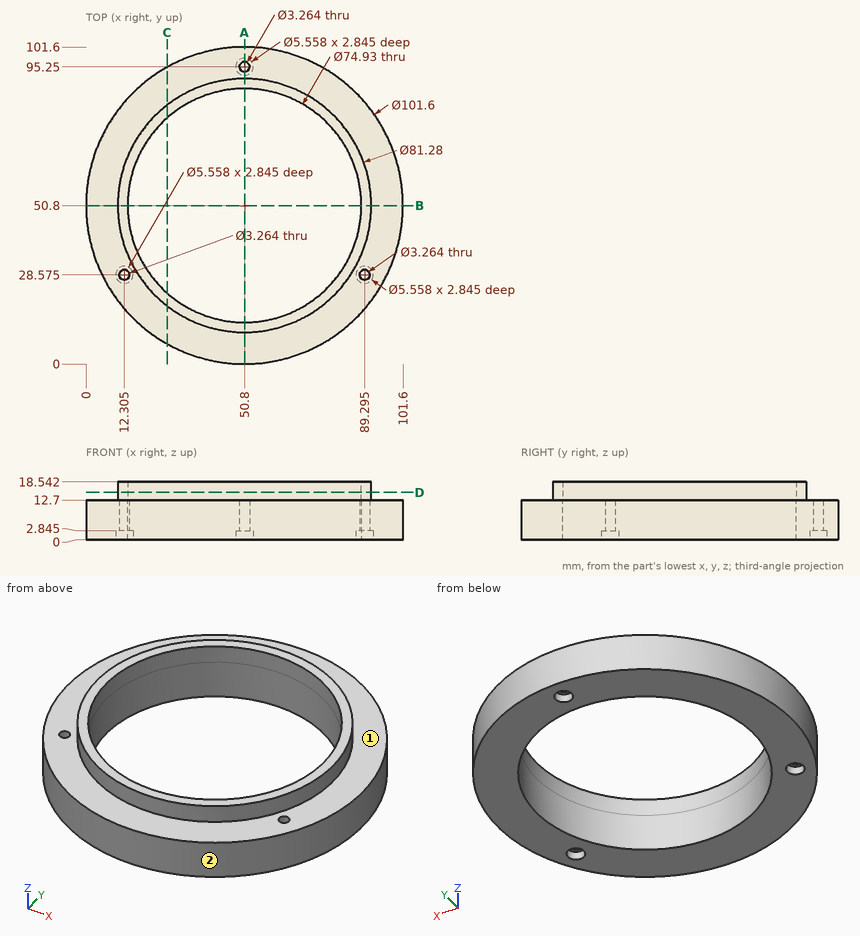
Source: three-view drawing plus pictorial views. Frame: mm from the lowest corner of the part. A direction names the side the tool comes from. Round coordinates to 2 decimals unless told otherwise and drop trailing zeros. Write each loop counter-clockwise with the first axis right and the second up, starting at its lowest first coordinate (ties: lowest second). Pieces come first, ordered by that corner, then holes. Notation, with made-up numbers: M 73,61.5 L 94,61.5 A19 ccw 94,98.5 Z; hole C -13.5,23 d6. An arc over 180 degrees is marked long. One line per item, written item: value. Start each with the question number.
Item 1: Pin query (flat end, axial travel): pin 1 (5 mm diameter, centred on y = 15.5, z = 7.5, fed in from +X); pin 2 (2 mm diameter, centred on y = 84, z = 14, fed in from +X) (1 decimal); pin 3 (4 mm diameter, centred on x = 89.29, y = 28.57, fed in from +Z). Return the tip coordinate at first contact, or that it passes through.
Item 2: Ray query, L1, parallel to Y at x = 50.8, z = 6.5 (1 decimal); L2, parallel to Y at x = 50.8, z = 16.85 (1 decimal); L3, parallel to Z at x = 21, y = 82. Return the intervals inside material, ascending. Write a range as from..to.
Item 3: Section query C-C (x = 26). Return the cut outline in (y, z) (1 decimal).
Item 4: Section query B-B (y = 50.8). Return the cut outline in (x, z) (1 decimal), plus the area to 3 significant figures.
Item 5: Set-up query: the marked faces 1 and 2. Return all of +Z, -Z, +X, -X, +Y, -Y with unobstructed straight access to the full face (end or side cutting, diameter ignored); none if empty.
Item 6: Section query D-D (z = 15.25). Return the cut outline in (x, y) (1 decimal).
Item 7: Section query A-A (x = 50.8). Return the cut outline in (y, z) (1 decimal), plus the area to 3 significant figures.
Result set:
1. pin 1: stops at x = 89.59
1. pin 2: stops at x = 75.6
1. pin 3: stops at z = 12.7
2. L1: y = 0..13.3, 88.3..93.6, 96.9..101.6
2. L2: y = 10.2..13.3, 88.3..91.4
2. L3: z = 0..12.7
3. outline: M 6.5,0 L 22.7,0 L 22.7,18.5 L 18.6,18.5 L 18.6,12.7 L 6.5,12.7 Z; M 78.9,0 L 95.1,0 L 95.1,12.7 L 83,12.7 L 83,18.5 L 78.9,18.5 Z
4. outline: M 0,0 L 13.3,0 L 13.3,18.5 L 10.2,18.5 L 10.2,12.7 L 0,12.7 Z; M 88.3,0 L 101.6,0 L 101.6,12.7 L 91.4,12.7 L 91.4,18.5 L 88.3,18.5 Z
4. area: 376 mm²
5. face 1: +Z
5. face 2: +Z, -Z
6. outline: C 50.8,50.8 d81.3; hole C 50.8,50.8 d74.9
7. outline: M 0,0 L 13.3,0 L 13.3,18.5 L 10.2,18.5 L 10.2,12.7 L 0,12.7 Z; M 88.3,0 L 92.5,0 L 92.5,2.8 L 93.6,2.8 L 93.6,12.7 L 91.4,12.7 L 91.4,18.5 L 88.3,18.5 Z; M 96.9,2.8 L 98,2.8 L 98,0 L 101.6,0 L 101.6,12.7 L 96.9,12.7 Z
7. area: 328 mm²
